Can you work these out from the drawing? Everything is in mm from the part's minimum corner. A direction names the side the tool comes from. Round coordinates to 2 decimals unless told otherwise and drop trailing zeros. Loops run counter-clockwise (first coordinate to the right, second up) from the corner with the lowest first, then second, coordinate; pieces in that order, holes last. Notation, with made-up numbers: (66.25, -15) -> (85.25, -15) arc R28 cw to (85.25, 8) -> close; hole circle Ø2 at (66.5, -15). An arc over 180 degrees is marked (long way). One line per item, written item: value.
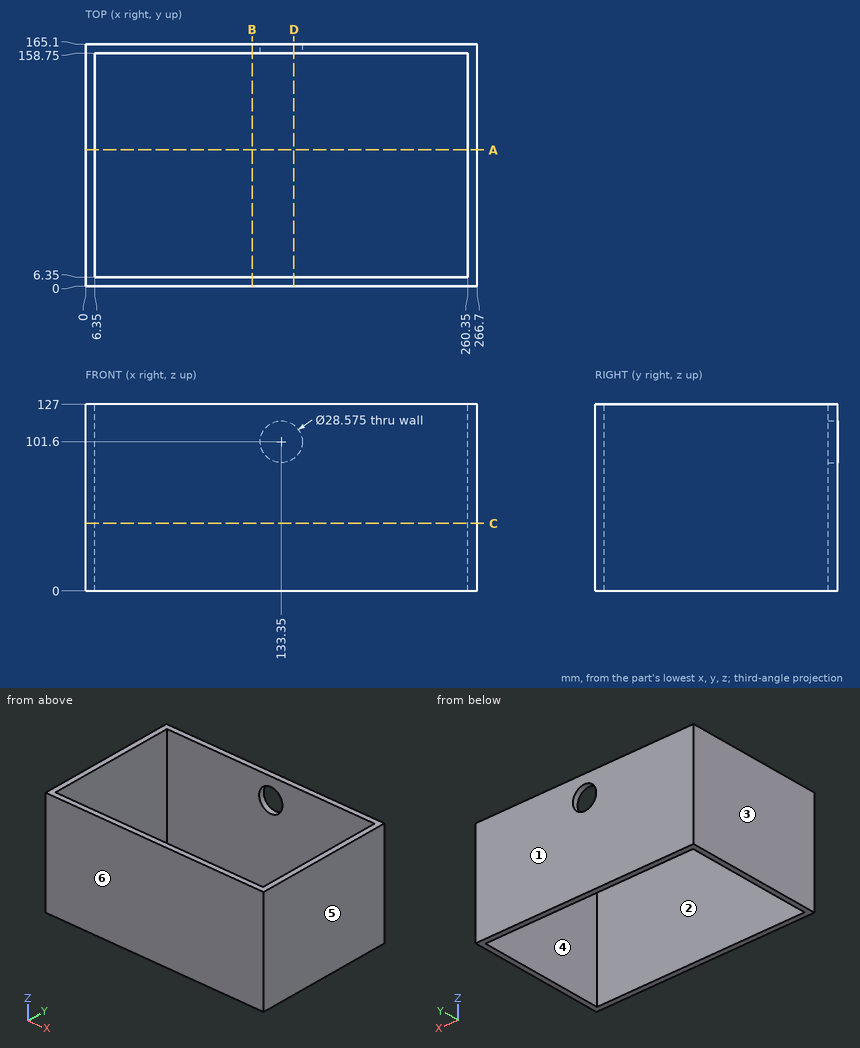
(1) If I drill on L1, parallel to X at y = 116.5, z = 26.5; L2, parallel to X at y = 162, z = 101; L3, parallel to Y at x = 160, z = 68, over which ranges is the centre line in solid material (lowest first)?
Recorded:
L1: 0 to 6.35, 260.35 to 266.7
L2: 0 to 119.08, 147.62 to 266.7
L3: 0 to 6.35, 158.75 to 165.1
(2) If we section it at B-B, the plane x = 113.5: Please give me the cut outline in (y, z), then the cut area to 3 significant figures.
Recorded:
outline: (0, 0) -> (6.35, 0) -> (6.35, 127) -> (0, 127) -> close; (158.75, 0) -> (165.1, 0) -> (165.1, 127) -> (158.75, 127) -> close
area: 1,610 mm²
(3) Thinking about a two-plate mould opening in X: for the marked faces 3, 4, 5 and 6, which applies, released by +X, released by -X, zero draft, split by the parting line, or undercut?
Recorded:
face 3: released by -X
face 4: undercut
face 5: released by +X
face 6: zero draft
(4) I'm going to push a flat-ended pin straight in: pin 1 Ø6 at (y, z) = (58, 101) entering from -X. Where does the tip first touch, or does it pass through?
Recorded:
pin 1: x = 0
(5) If we section it at D-D, the plane x = 142: Please give me the cut outline in (y, z), then the cut area to 3 significant figures.
Recorded:
outline: (0, 0) -> (6.35, 0) -> (6.35, 127) -> (0, 127) -> close; (158.75, 0) -> (165.1, 0) -> (165.1, 90.23) -> (158.75, 90.23) -> close; (158.75, 112.97) -> (165.1, 112.97) -> (165.1, 127) -> (158.75, 127) -> close
area: 1,470 mm²
(6) If we section it at A-A, the plane y = 93: Please give me the cut outline in (x, z), then the cut area to 3 significant figures.
Recorded:
outline: (0, 0) -> (6.35, 0) -> (6.35, 127) -> (0, 127) -> close; (260.35, 0) -> (266.7, 0) -> (266.7, 127) -> (260.35, 127) -> close
area: 1,610 mm²
(7) If we section it at C-C, the plane z = 46: Please give me the cut outline in (x, y), then the cut area to 3 significant figures.
Recorded:
outline: (0, 0) -> (266.7, 0) -> (266.7, 165.1) -> (0, 165.1) -> close; hole (6.35, 6.35) -> (260.35, 6.35) -> (260.35, 158.75) -> (6.35, 158.75) -> close
area: 5,320 mm²
(8) For the marked faces 1 and 2, which set-ups out of +Z, -Z, +X, -X, +Y, -Y let a thin tool reach every point of the face, with its end or its side?
Recorded:
face 1: +Z, -Z, +X, -X, +Y
face 2: +Z, -Z
